Autodesk Inventor part; units mm, degrees
ref_plane "YZ Plane" through (0, 0, 0) normal (1, 0, 0) x (0, 1, 0)
ref_plane "XZ Plane" through (0, 0, 0) normal (0, 1, 0) x (-1, 0, 0)
ref_plane "XY Plane" through (0, 0, 0) normal (0, 0, 1) x (1, 0, 0)
sketch "Эскиз1" plane through (0, 0, 0) normal (0, 0, 1) x (1, 0, 0)
  line L0 (30, 30) -> (0, 30)
  line L1 (0, 30) -> (0, 0)
  line L2 (30, 30) -> (30, 22)
  line L3 (5, 0) -> (5, 27)
  line L4 (5, 27) -> (27, 27)
  line L5 (27, 27) -> (27, 22)
  line L6 (0, 0) -> (5, 0)
  line L7 (27, 22) -> (30, 22)
  dimension "d0" = 30
  dimension "d2" = 30
  dimension "d5" = 5
  dimension "d6" = 8
  dimension "d15" = 3
  dimension "d16" = 3
  dimension "d17" = 5
extrude "Выдавливание1" add sketch "Эскиз1" against normal blind 80
sketch "Эскиз2" plane through (0, 0, 0) normal (-1, 0, 0) x (0, 0, 1)
  line L0 (0, 30) -> (-80, 30)
  line L1 (-70, 30) -> (-70, 0) construction
  line L2 (0, 0) -> (-80, 0)
  circle A0 centre (-70, 15) radius 3 construction
  line L3 (-68.2679, 18) -> (-66.5359, 15)
  line L4 (-66.5359, 15) -> (-68.2679, 12)
  line L5 (-68.2679, 12) -> (-71.7321, 12)
  line L6 (-71.7321, 12) -> (-73.4641, 15)
  line L7 (-73.4641, 15) -> (-71.7321, 18)
  line L8 (-71.7321, 18) -> (-68.2679, 18)
  line L9 (-80, 0) -> (-80, 30)
  line L10 (0, 30) -> (-80, 30)
  point P0 (-70, 18)
  dimension "d9" = 6
  dimension "d30" = 10
extrude "Выдавливание2" cut sketch "Эскиз2" against normal blind 4
sketch "Эскиз3" plane through (4, 0, 0) normal (-1, 0, 0) x (0, 0, 1)
  line L0 (-71.7321, 18) -> (-68.2679, 18)
  line L1 (-70, 18) -> (-70, 12) construction
  line L2 (-68.2679, 12) -> (-71.7321, 12)
  circle A0 centre (-70, 15) radius 1.75
  point P0 (0, 0)
  dimension "d18" = 3.5
extrude "Выдавливание3" cut sketch "Эскиз3" against normal up to next
ref_plane "РабПлоскость1" through (0, 0, -40) normal (0, 0, -1) x (-1, 0, 0)
sketch "Эскиз4" plane through (0, 0, -40) normal (0, 0, -1) x (-1, 0, 0)
  arc A0 (-20.9616, 74.2788) -> (-39.6825, 67.5) centre (-30, 70) ccw
  line L0 (-30, 30) -> (-30, 22)
  line L1 (-30, 30) -> (-39.6825, 67.5)
  line L2 (0, 30) -> (0, 0)
  line L3 (0, 30) -> (-20.9616, 74.2788)
  circle A1 centre (-30, 70) radius 1.75
  line L4 (-30, 22) -> (-30, 30)
  line L5 (-30, 30) -> (0, 30)
  line L6 (-30, 22) -> (-27, 22)
  dimension "d21" = 20
  dimension "d22" = 3.5
  dimension "d31" = 30
  dimension "d32" = 40
extrude "Выдавливание4" add sketch "Эскиз4" along normal mid plane 10
fillet "Сопряжение1" radius 5 2 edges at (15, 30, -45) (15, 30, -35)
mirror "Зеркальное отражение1" about plane through (0, 0, -40) normal (0, 0, -1) of "Выдавливание2", "Выдавливание3"
sketch "Эскиз5" plane through (5, 0, 0) normal (1, 0, 0) x (0, 0, -1)
  point P0 (0, 0)
equation "\"d6\" = d5 + d4"
properties part number "holder"
Geometry: final body of the model. Coordinates: model frame, mm. A direction names the side the tool comes from. Coordinates: 2 decimals unless noted, no trailing zeros. Order: outer loops, then holes, each group sorted by start corner. A loop starts at its lowest first (then second) coordinate and runs counter-clockwise, first axis right, second up. Notation, with made-up numbers: (37.5, 40.5) -> (74.5, 40.5) arc R17 ccw to (74.5, 60.5) -> close; hole circle Ø7 at (60, 54.25). An arc over 180 degrees is marked (long way). Write each question's results on one line, items separated by ' | '. Start each with the question number.
1) Cut plane D-D, the plane y = 55.5. Output: boundary loops of the cut face in (x, z), and give its area (3 significant figures).
2) Material intervals for line 1 along X through (y, z) = (24, -40); line 2 along Y through (x, z) = (28, -6); line 3 along Y through (x, z) = (11, -26.5), sorted ascending.
3) Cut plane C-C, the plane z = -64. Output: boundary loops of the cut face in (x, y), and give its area (3 significant figures).
4) Cut plane A-A, the plane z = -10. Output: boundary loops of the cut face in (x, y).
5) Cut plane B-B, the plane y = 70. Output: boundary loops of the cut face in (x, z).
6) Mould query, pull axis Y, two halves, no side actions, for faces 1 (the cylindrical face through (31.39, 71.06, -39.93)), 2 (the flat face through (15, 30, -15)), 3 (the flat face through (28, 22, -39)), 4 (the flat face through (26, 58, -35)). Classes: released by +Y, released by -Y, zero draft, split by the parting line, or undercut.
7) First-contact query: pin 1 (1 mm diameter, centred on x = 2, z = -9, fed in from +Y); pin 2 (10 mm diameter, centred on x = 8.5, y = 44, fed in from +Z); pin 3 (2.5 mm diameter, centred on x = 28, z = -27, fed in from -Y). Flat tips, straight axial feed; report the tip coordinate or a pass-through.
8) Set-up query: faces 5 (the flat face through (4, 13.7, -8.5)), 6 (the flat face through (16, 27, -39)), 7 (the flat face through (4, 18, -80)). Return all of +Z, -Z, +X, -X, +Y, -Y with unobstructed straight access to the full face (end or side cutting, diameter ignored); none if empty.
Checks:
1) outline: (12.07, -45) -> (36.58, -45) -> (36.58, -35) -> (12.07, -35) -> close | area: 245 mm^2
2) line 1: 0 to 5, 27 to 30 | line 2: 22 to 30 | line 3: 27 to 30
3) outline: (0, 0) -> (5, 0) -> (5, 27) -> (27, 27) -> (27, 22) -> (30, 22) -> (30, 30) -> (0, 30) -> close | area: 240 mm^2
4) outline: (0, 0) -> (5, 0) -> (5, 13.25) -> (4, 13.25) -> (4, 12) -> (0, 12) -> close; (0, 18) -> (4, 18) -> (4, 16.75) -> (5, 16.75) -> (5, 27) -> (27, 27) -> (27, 22) -> (30, 22) -> (30, 30) -> (0, 30) -> close
5) outline: (18.94, -45) -> (28.25, -45) -> (28.25, -35) -> (18.94, -35) -> close; (31.75, -45) -> (40, -45) -> (40, -35) -> (31.75, -35) -> close
6) face 1: undercut | face 2: released by +Y | face 3: released by -Y | face 4: zero draft
7) pin 1: y = 30 | pin 2: z = -35 | pin 3: y = 22
8) face 5: -X | face 6: +Z, -Z, -Y | face 7: -Z, +X, -X, +Y, -Y
